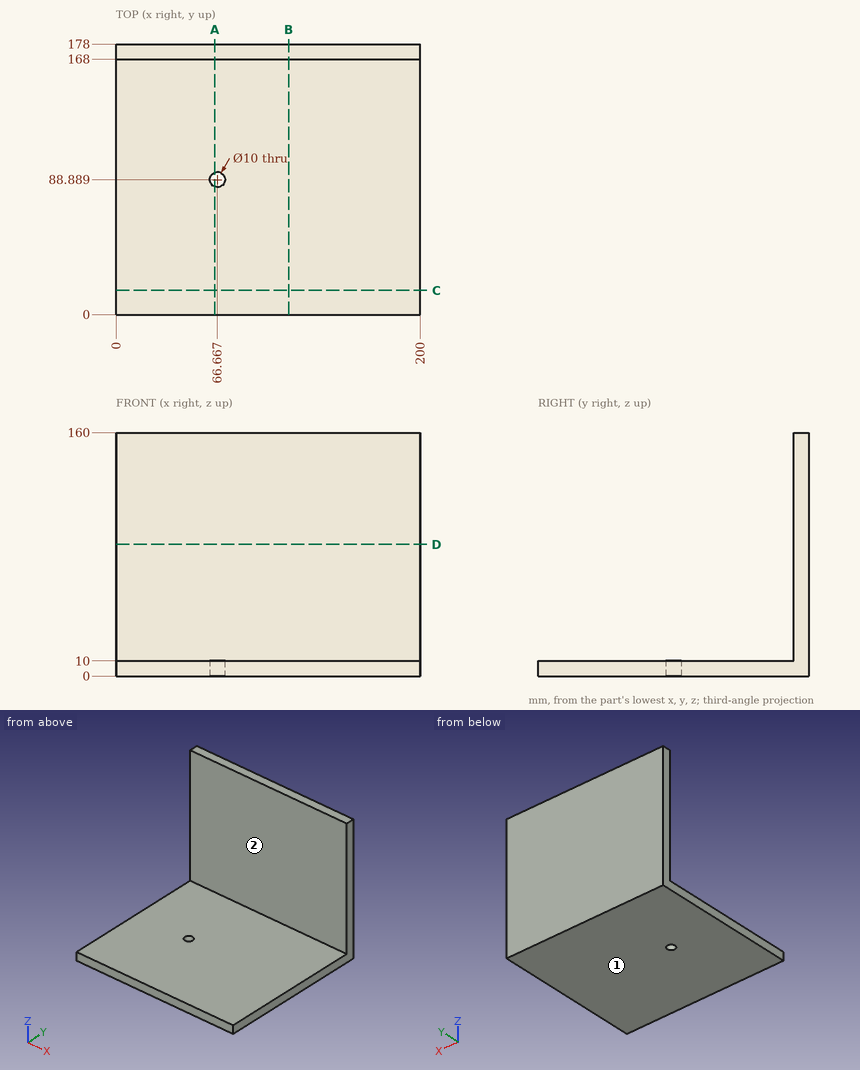
The drawing under review shows one solid part. Ordinate dimensions are in mm from its lowest x, y, z. A direction names the side the tool comes from. Coordinates: 2 decimals unless noted, no trailing zeros. Order: outer loops, then holes, each group sorted by start corner. A loop starts at its lowest first (then second) coordinate and runs counter-clockwise, first axis right, second up. Notation, with made-up numbers: (43.25, 25.25) -> (55.25, 25.25) arc R19 ccw to (55.25, 49.25) -> close; hole circle Ø1 at (50, 30). An arc over 180 degrees is marked (long way). Use CSV: the item, a comma, the result in double quotes. Start each with the question number.
Item 1: Insertion check: pin 1 (10 mm diameter, centred on x = 113, y = 67, fed in from +Z). The pin has a flat end and moves straight along its axis. Give the tip position at first contact, or say it passes through.
Item 2: We need section B-B, the plane x = 113.5. Give the boundary of the cut face in (y, z).
Item 3: Wall thickness on probe 1 along Z at (x, y) = (69, 149); probe 2 along Y at (x, z) = (27, 116.5): over which ranges is each line inside the solid? List them lowest first.
Item 4: We need section A-A, the plane x = 65. Give the boundary of the cut face in (y, z) (1 decimal).
Item 5: For the marked faces 1 and 2, list the 3-axis set-ups (+Z, -Z, +X, -X, +Y, -Y) from which the entire face can be reached by the end or side of a thin tool; tool diameter is ignored.
Item 6: We need section C-C, the plane y = 16. Give the boundary of the cut face in (x, z).
Item 7: We need section D-D, the plane z = 86.5. Give the boundary of the cut face in (x, y).
Derived:
1,pin 1,"stops at z = 10"
2,outline,"(0, 0) -> (178, 0) -> (178, 160) -> (168, 160) -> (168, 10) -> (0, 10) -> close"
3,probe 1,"z = 0 to 10"
3,probe 2,"y = 168 to 178"
4,outline,"(0, 0) -> (84.2, 0) -> (84.2, 10) -> (0, 10) -> close; (93.6, 0) -> (178, 0) -> (178, 160) -> (168, 160) -> (168, 10) -> (93.6, 10) -> close"
5,face 1,"-Z, +X, -X, +Y, -Y"
5,face 2,"+Z, +X, -X, -Y"
6,outline,"(0, 0) -> (200, 0) -> (200, 10) -> (0, 10) -> close"
7,outline,"(0, 168) -> (200, 168) -> (200, 178) -> (0, 178) -> close"
